Read the model definition and answer for the solid it produces. Units are mm, in the model's axes. A direction names the side the tool comes from. Round coordinates to 2 decimals unless told otherwise and drop trailing zeros. Loops run counter-clockwise (first coordinate to the right, second up) from the corner with the lowest first, then second, coordinate; pieces in that order, holes last. Notation, with made-up numbers: (-8, 58) -> (35, 58) arc R30 ccw to (35, 96) -> close; hole circle Ø4 at (-29.5, -13). An arc over 180 degrees is marked (long way). Put each result on its own line as item: value.
Autodesk Inventor part; units mm, degrees
ref_plane "YZ Plane" through (0, 0, 0) normal (1, 0, 0) x (0, 1, 0)
ref_plane "XZ Plane" through (0, 0, 0) normal (0, 1, 0) x (-1, 0, 0)
ref_plane "XY Plane" through (0, 0, 0) normal (0, 0, 1) x (1, 0, 0)
sketch "Sketch1" plane through (0, 0, 0) normal (0, 0, 1) x (1, 0, 0)
  line L0 (-7.1438, 20.6375) -> (-9.525, 20.6375)
  line L1 (-9.525, 20.6375) -> (-9.525, 4.0656)
  line L2 (-12.7, 0) -> (0, 0)
  line L3 (0, -4.6495) -> (0, 24.852)
  line L4 (-7.1438, 20.6375) -> (-7.1437, 8.8537)
  line L5 (-6.3504, 7.4791) -> (0, 3.81)
  line L6 (0, 3.81) -> (0, 0)
  arc A0 (-10.5933, 2.5654) -> (-9.525, 4.0656) centre (-11.1125, 4.0656) ccw
  arc A1 (-10.5933, 2.5654) -> (-12.7, 0) centre (-9.5549, -0.435) ccw
  arc A2 (-7.1437, 8.8537) -> (-6.3504, 7.4791) centre (-5.5563, 8.8537) ccw
  point P0 (-9.525, 3.175)
  point P1 (-7.1437, 7.9375)
  dimension "d0" = 20.6375
  dimension "d1" = 19.05
  dimension "d2" = 14.2875
  dimension "d3" = 12.7
  dimension "d4" = 3.175
  dimension "d5" = 25.4
  dimension "d6" = 1.5875
  dimension "d7" = 3.175
  dimension "d8" = 3.81
  dimension "d10" = 1.5875
revolve "Revolution1" add sketch "Sketch1" angle 360 about axis through (0, -10, 0) along (0, 1, 0)
chamfer "Chamfer1" distance 0.127 angle 45 2 edges at (9.525, 20.6375, 0) (7.1438, 20.6375, 0)
sketch "Sketch2" plane through (0, 20.6375, 0) normal (0, 1, 0) x (1, 0, 0)
  line L0 (1.5875, 9.6188) -> (1.5875, 6.8545)
  line L1 (1.5875, 6.8545) -> (-1.5875, 6.8545) construction
  line L2 (-1.5875, 6.8545) -> (-1.5875, 9.6188)
  line L3 (0, 17.78) -> (0, -17.78) construction
  arc A0 (1.5875, 9.4869) -> (-1.5875, 9.4869) centre (0, 0) ccw
  arc A1 (1.5875, 6.9651) -> (-1.5875, 6.9651) centre (0, 0) ccw
  dimension "d14" = 3.175
  dimension "d15" = 1.5875
extrude "Extrusion1" cut sketch "Sketch2" against normal blind 9.525
pattern_circular "Circular Pattern1" count 4 over 360 about axis through (0, -10, 0) along (0, 1, 0) of "Extrusion1"
equation "\"d15\" = 0.5 * d14"
properties part number "Disco de Apriete" material "Aluminum 6061-AHC"
Item 1: Flat-ended cylindrical pins translate along their axes: pin 1 Ø0.7 at (y, z) = (18, 7.5) entering from +X; pin 2 Ø1.2 at (x, y) = (-8, 15) entering from -Z; pin 3 Ø12 at (y, z) = (11, 1.5) entering from -X (3 decimals); pin 4 Ø1 at (x, z) = (10, 9) entering from +Y. Find the tip coordinate at first contact, or state that the pin passes through.
Derived:
pin 1: stops at x = 6.29
pin 2: stops at z = -6
pin 3: stops at x = -9.525
pin 4: passes through
Item 2: For a pull along Z with two mould halves and no side action, classify faces 4 (the cylindrical face through (-6.599, 14.601, 2.736)), 5 (the flat face through (-1.588, 16, 8)) as pulls with the +Z half, pulls with the -Z half, needs draft (parallel to the pull), parting line crosses it, or undercut.
Derived:
face 4: undercut
face 5: needs draft
Item 3: The part is cut by section B-B (y = 7). Determine the outline of the cut face in (x, z) (3 decimals).
Derived:
outline: circle Ø19.05 at (0, 0); hole circle Ø11.042 at (0, 0)
Item 4: The part is cut by section A-A (y = 10.25). Determine the outline of the cut face in (x, z) (3 decimals).
Derived:
outline: circle Ø19.05 at (0, 0); hole circle Ø14.288 at (0, 0)
Item 5: Which of the six approach directions +Z, -Z, +X, -X, +Y, -Y give full straight-line access (tool end or side, diameter ignored) to faces 1 (the flat face through (-5.4, 20.638, 5.5)), 2 (the flat face through (1.588, 16, 8)), 3 (the flat face through (8, 11.112, 0))?
Derived:
face 1: +Z, -Z, +X, -X, +Y
face 2: +Z, -Z, +Y
face 3: +X, -X, +Y
Item 6: Find the intervals of material crossed by line 1 along X through (y, z) = (19.25, 3.75); line 2 along X through (y, z) = (8, 4.25); line 3 along Z through (x, y) = (-7.5, 13), in increasing order.
Derived:
line 1: x = -8.76 to -6.08, 6.08 to 8.76
line 2: x = -8.52 to -5.43, 5.43 to 8.52
line 3: z = -5.87 to -1.59, 1.59 to 5.87
